Verification items for the finished model (mm, model axes). Face numbers are marked on the shaded views. A direction names the side the tool comes from. Round coordinates to 2 decimals unless told otherwise and drop trailing zeros. Loops run counter-clockwise (first coordinate to the right, second up) from the corner with the lowest first, then second, coordinate; pieces in that order, holes last. Notation, with made-up numbers: (50, -5.75) -> (56, -5.75) arc R24 ccw to (56, 5.25) -> close; hole circle Ø8 at (0, 25.5). An arc over 180 degrees is marked (long way). Use a Markdown table: item, result. Add a question column.
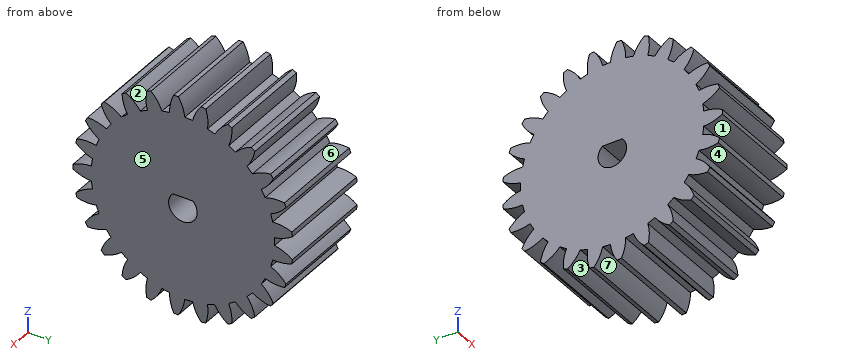
```python
from build123d import *

# Parameters (mm, degrees)
BASPROSKE_W         = 12
BASPROSKE_H         = 13.5
TOOTHCUT_DEPTH      = 23.549944568
TEETHCUTS_COUNT     = 25
TEETHCUTS_ANGLE     = 345.6
BORSKE_R            = 1.5
BORE_DEPTH          = 50.0000508
CUT_EXTRUDE1_DEPTH  = 23.542777009
BOSS_EXTRUDE2_DEPTH = 12


with BuildPart() as part:
    # BasProSke → Base-Revolve (revolve)
    with BuildSketch(Plane(origin=(0, 0, 0), x_dir=(1, 0, 0), z_dir=(0, 1, 0)), mode=Mode.PRIVATE) as base_revolve_sk:
        with Locations((6, 6.75)):
            Rectangle(BASPROSKE_W, BASPROSKE_H)
    revolve(base_revolve_sk.sketch.rotate(Axis((-10, 0, 0), (1, 0, 0)), 180), axis=Axis((-10, 0, 0), (1, 0, 0)))

    # TooCutSke → ToothCut (cut, through all)
    with BuildSketch(Plane(origin=(0, 0, 0), x_dir=(0, 0, -1), z_dir=(1, 0, 0))):
        with BuildLine():
            ThreePointArc((0.480087995, 11.238750665), (0, 11.249), (-0.480087995, 11.238750665))
            ThreePointArc((-0.480087995, 11.238750665), (-0.821124963, 12.40220054), (-1.432168974, 13.449361962))
            ThreePointArc((-1.432168974, 13.449361962), (0, 13.5254), (1.432168974, 13.449361962))
            ThreePointArc((1.432168974, 13.449361962), (0.821124963, 12.40220054), (0.480087995, 11.238750665))
        make_face()
    toothcut = extrude(amount=TOOTHCUT_DEPTH, mode=Mode.SUBTRACT)

    # TeethCuts: ToothCut ×25 about axis
    teethcuts_axis = Axis((-10, 0, 0), (1, 0, 0))
    for i in range(1, TEETHCUTS_COUNT):
        add(toothcut.rotate(teethcuts_axis, i * TEETHCUTS_ANGLE / (TEETHCUTS_COUNT - 1)), mode=Mode.SUBTRACT)

    # BorSke → Bore (cut, symmetric)
    with BuildSketch(Plane(origin=(0, 0, 0), x_dir=(0, 0, -1), z_dir=(1, 0, 0))):
        with Locations(Location((0, 0, 0), (0, 0, 180))):
            Circle(BORSKE_R)
    extrude(amount=BORE_DEPTH, both=True, mode=Mode.SUBTRACT)

    # Sketch1 → Cut-Extrude1 (cut, through all)
    with BuildSketch(Plane(origin=(12, 0, 0), x_dir=(0, 0, -1), z_dir=(1, 0, 0))):
        with BuildLine():
            Line((-1.25, 1.224744871), (-1.25, -1.224744871))
            ThreePointArc((-1.25, -1.224744871), (1.75, 0), (-1.25, 1.224744871))
        make_face()
    extrude(amount=-CUT_EXTRUDE1_DEPTH, mode=Mode.SUBTRACT)

    # Sketch1<4> → Boss-Extrude2 (add, through all)
    with BuildSketch(Plane(origin=(12, 0, 0), x_dir=(0, 0, -1), z_dir=(1, 0, 0))):
        with BuildLine():
            Line((-1.25, -0.829156198), (-1.25, 0.829156198))
            ThreePointArc((-1.25, 0.829156198), (-1.5, 0), (-1.25, -0.829156198))
        make_face()
    extrude(amount=-BOSS_EXTRUDE2_DEPTH)


solid = part.part
```
1) Release check for a two-part mould opening along Z. For the marked faces 5, 6 and 7 record: released by +Z, released by -Z, zero draft, split by the parting line, or undercut.
2) Sectioned sample at B-B on y = 7.5. Enter the section's corners in (x, z).
3) Go/stop test with flat-tipped pins: pin 1 (3 mm diameter, centred on x = 10, z = 4.5, fed in from +Y); pin 2 (3 mm diameter, centred on x = 3.5, y = 8.5, fed in from -Z); pin 3 (2 mm diameter, centred on x = 6, y = 8.5, fed in from +Z). Record where each tip stops, or that it passes through.
4) Access from +Z, -Z, +X, -X, +Y, -Y to the whole of each face (thin tool, end or side, straight path). Record for the marked faces 1, 2, 3 and 4.
5) Sectioned sample at A-A on y = 0.75. Enter the section's corners in (x, z), then the cut area to 3 significant figures.
6) Thickness scan on line 1 (Y direction, x = 4.75, z = 0); line 2 (Y direction, x = 5.5, z = -10.5); line 3 (Z direction, x = 9.5, y = 10.5). Record the ranges inside material, lowest first.
Geometry results:
| question | item | result |
|---|---|---|
| 1 | face 5 | zero draft |
| 1 | face 6 | undercut |
| 1 | face 7 | released by -Z |
| 2 | outline | (0, -10.14) -> (12, -10.14) -> (12, 10.14) -> (0, 10.14) -> close |
| 3 | pin 1 | y = 12.65 |
| 3 | pin 2 | z = -10.58 |
| 3 | pin 3 | z = 10.58 |
| 4 | face 1 | +X, -X, -Y |
| 4 | face 2 | +Z, +X, -X |
| 4 | face 3 | -Z, +X, -X |
| 4 | face 4 | +X, -X |
| 5 | outline | (0, -11.22) -> (12, -11.22) -> (12, -1.58) -> (0, -1.58) -> close; (0, 1.25) -> (12, 1.25) -> (12, 11.22) -> (0, 11.22) -> close |
| 5 | area | 235 mm^2 |
| 6 | line 1 | -13.5 to -1.75, 1.75 to 11.25 |
| 6 | line 2 | -7.38 to -5.65, -4.38 to 5.87, 8.19 to 8.49 |
| 6 | line 3 | -8.12 to -6.73, -5.12 to 5.12, 6.73 to 8.12 |
